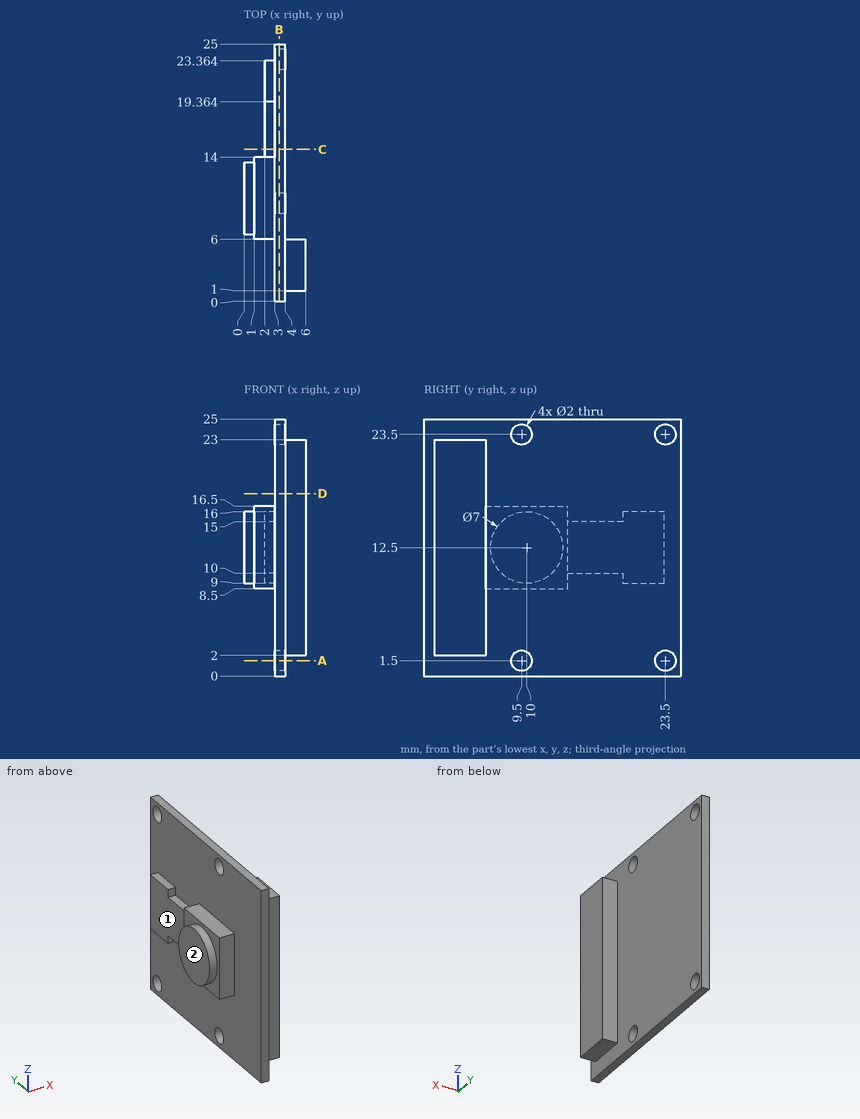
For this review, use the dimensioned drawing (mm, ordinates from the lowest corner) and the shaded views. A direction names the side the tool comes from. Round coordinates to 2 decimals unless told otherwise and drop trailing zeros. Order: outer loops, then holes, each group sorted by start corner. A loop starts at its lowest first (then second) coordinate and runs counter-clockwise, first axis right, second up. Notation, with made-up numbers: M -23,-19 L 25,-19 A16 cw 25,-14 Z; hole C -14,-40 d1. An arc over 180 degrees is marked long. Use a Markdown table: item, result. Add a question column.
Item 1: Add section C-C, the plane y = 14.75. Give the boundary of the cut face in (x, z), then the cut area to 3 significant figures.
Item 2: Tool access review of the marked faces 1 and 2: name each direction out of +Z, -Z, +X, -X, +Y, -Y from which nothing blocks a thin tool from reaching the whole face with its end or side.
Item 3: Add section B-B, the plane x = 3.4. Give the boundary of the cut face in (y, z), then the cut area to 3 significant figures.
Item 4: Add section D-D, the plane z = 17.75. Give the boundary of the cut face in (x, y).
Item 5: Add section A-A, the plane z = 1.5. Give the boundary of the cut face in (x, y).
Item 6: To check wall thickness, follow line 1 along Y through (x, z) = (3.6, 23.5); line 2 along Y through (x, z) = (4.55, 22.5); line 3 along X through (y, z) = (14, 5.25). State the ranges of each line that lie inside material, in increasing order.
Item 7: Insertion check: pin 1 (3 mm diameter, centred on y = 9.5, z = 1.5, fed in from -X); pin 2 (0.6 mm diameter, centred on x = 2.5, z = 12.5, fed in from -Y); pin 3 (8 mm diameter, centred on y = 15.5, z = 5, fed in from +X). Each pin has a flat end and moves straight along its axis. Give the tip position at first contact, or say it passes through.
Geometry results:
| question | item | result |
|---|---|---|
| 1 | outline | M 2,10 L 3,10 L 3,0 L 4,0 L 4,25 L 3,25 L 3,15 L 2,15 Z |
| 1 | area | 30.0 mm² |
| 2 | face 1 | +Z, -Z, -X, +Y |
| 2 | face 2 | +Z, -Z, -X, +Y, -Y |
| 3 | outline | M 0,0 L 25,0 L 25,25 L 0,25 Z; hole C 9.5,1.5 d2; hole C 9.5,23.5 d2; hole C 23.5,1.5 d2; hole C 23.5,23.5 d2 |
| 3 | area | 612 mm² |
| 4 | outline | M 3,0 L 4,0 L 4,1 L 6,1 L 6,6 L 4,6 L 4,25 L 3,25 Z |
| 5 | outline | M 3,0 L 4,0 L 4,8.5 L 3,8.5 Z; M 3,10.5 L 4,10.5 L 4,22.5 L 3,22.5 Z; M 3,24.5 L 4,24.5 L 4,25 L 3,25 Z |
| 6 | line 1 | y = 0 to 8.5, 10.5 to 22.5, 24.5 to 25 |
| 6 | line 2 | y = 1 to 6 |
| 6 | line 3 | x = 3 to 4 |
| 7 | pin 1 | stops at x = 3 |
| 7 | pin 2 | stops at y = 6 |
| 7 | pin 3 | stops at x = 4 |
